Autodesk Fusion 360 part; units mm, degrees
sketch "草图1" plane through (0, 0, 0) normal (0, 1, 0) x (1, 0, 0)
  line L0 (0, -75) -> (0, 75) construction
  line L1 (0, 20) -> (13, 20)
  line L2 (14, 19) -> (14, 5.8348)
  line L3 (16, 3.8348) -> (27, 3.8348)
  line L4 (27, 3.8348) -> (27, -12.1652)
  line L5 (0, 20) -> (0, -15)
  arc A0 (0, -15) -> (27, -12.1652) centre (0, 115) ccw
  arc A1 (14, 5.8348) -> (16, 3.8348) centre (16, 5.8348) ccw
  line L6 (13, 20) -> (14, 19)
  point P0 (14, 20)
  dimension "d1" = 20
  dimension "d2" = 14
  dimension "d3" = 16
  dimension "d4" = 35
  dimension "d5" = 130
  dimension "d6" = 27
  dimension "d7" = 2
  dimension "d8" = 1
  dimension "d9" = 45
revolve "旋转1" add sketch "草图1" angle 360 about axis through (0, 0, 75) along (0, 0, -1)
sketch "草图2" plane through (0, 0, 0) normal (0, 0, 1) x (1, 0, 0)
  circle A0 centre (0, 0) radius 27
  circle A1 centre (0, 0) radius 22 construction
  arc A2 (-9.8452, 25.141) -> (9.8452, 25.141) centre (0, 39) ccw
  line L0 (0, 40) -> (0, -45) construction
  arc A3 (-26.6954, 4.0443) -> (-16.8501, 21.0967) centre (-33.775, 19.5) ccw
  arc A4 (-16.8501, -21.0967) -> (-26.6954, -4.0443) centre (-33.775, -19.5) ccw
  arc A5 (9.8452, -25.141) -> (-9.8452, -25.141) centre (0, -39) ccw
  arc A6 (26.6954, -4.0443) -> (16.8501, -21.0967) centre (33.775, -19.5) ccw
  arc A7 (16.8501, 21.0967) -> (26.6954, 4.0443) centre (33.775, 19.5) ccw
  dimension "d11" = 54
  dimension "d12" = 44
  dimension "d13" = 17
  dimension "d15" = 360
extrude "拉伸1" cut sketch "草图2" along normal through all and the other way through all contours A0 A2 A3 A4 A5 A6 A7 keep common part
hole "孔1" at (0, 0, -20) direction (0, 0, 1) diameter 10 depth 20 tip angle 118
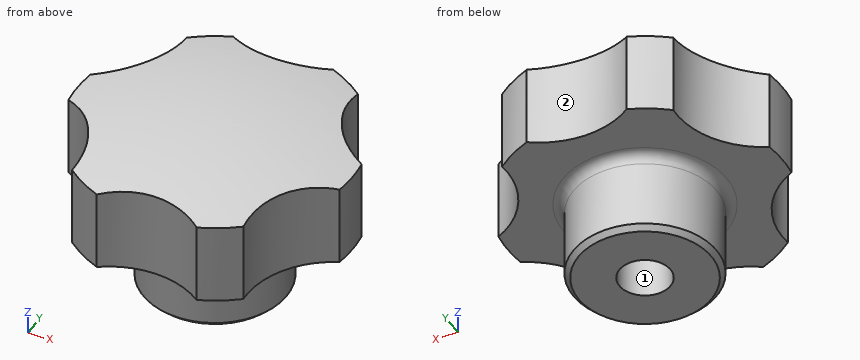
For this review, take the finished solid that the model builds, in its own axes (mm). Face numbers are marked on the shaded views. A direction names the side the tool comes from. Give positions to 0.01 mm unless a question says otherwise; leave off trailing zeros. Write each loop counter-clockwise with the first axis right and the second up, starting at its lowest first coordinate (ties: lowest second). Pieces come first, ordered by that corner, then holes.
Item 1: Wall thickness on probe 1 along Y at (x, z) = (0, -13); probe 2 along Z at (x, y) = (2, 16): over which ranges is each line inside the solid? List them lowest first.
Item 2: Take a section at A-A (z = 6). Give the boundary of the cut face in (x, y).
Item 3: Machinability: for the marked faces 1 and 2, which of the approach directions +Z, -Z, +X, -X, +Y, -Y give a long, thin tool a straight path to every point of the face, cutting with its end or side? Answer none if there is none.
Item 4: Insertion check: P1, Ø3, axis at x = -21.5, y = 4, coming from the -Z side; P2, Ø1, axis at x = -17, y = -17, coming from the +Z side; P3, Ø10, axis at y = 8, z = -16.5, coming from the +X side. Each pin has a flat end and moves straight along its axis. Give the tip position at first contact, or say it passes through.
Item 5: Take a section at B-B (z = -12). Give the boundary of the cut face in (x, y).
Established:
1. probe 1: y = -14 to -5, 5 to 14
1. probe 2: z = -3.83 to 14
2. outline: (-26.7, -4.04) arc R17 cw to (-16.85, -21.1) arc R27 ccw to (-9.85, -25.14) arc R17 cw to (9.85, -25.14) arc R27 ccw to (16.85, -21.1) arc R17 cw to (26.7, -4.04) arc R27 ccw to (26.7, 4.04) arc R17 cw to (16.85, 21.1) arc R27 ccw to (9.85, 25.14) arc R17 cw to (-9.85, 25.14) arc R27 ccw to (-16.85, 21.1) arc R17 cw to (-26.7, 4.04) arc R27 ccw to start
3. face 1: -Z
3. face 2: +Z, -Z, +Y
4. P1: stops at z = -3.83
4. P2: stops at z = 12.85
4. P3: stops at x = 13.67
5. outline: circle Ø28 at (0, 0); hole circle Ø10 at (0, 0)
